Design review of the part built by this model. Coordinates are the model's own, in mm. Give positions to 0.01 mm unless a question says otherwise; leave off trailing zeros. Write each loop counter-clockwise with the first axis right and the second up, starting at its lowest first coordinate (ties: lowest second). Pieces come first, ordered by that corner, then holes.
Autodesk Inventor part; units mm, degrees
ref_plane "YZ Plane" through (0, 0, 0) normal (1, 0, 0) x (0, 1, 0)
ref_plane "XZ Plane" through (0, 0, 0) normal (0, 1, 0) x (-1, 0, 0)
ref_plane "XY Plane" through (0, 0, 0) normal (0, 0, 1) x (1, 0, 0)
sketch "Boceto1" plane through (0, 0, 0) normal (0, 0, 1) x (1, 0, 0)
  line L0 (70, -75) -> (-70, -75)
  line L1 (-70, -75) -> (-70, 75)
  line L2 (-70, 75) -> (70, 75)
  line L3 (70, 75) -> (70, -75)
  line L4 (70, -75) -> (-70, 75) construction
  line L5 (-70, -75) -> (70, 75) construction
  point P0 (0, 0)
  dimension "d0" = 140
  dimension "d1" = 150
extrude "Extrusión1" add sketch "Boceto1" along normal blind 6
sketch "Boceto2" plane through (0, 0, 6) normal (0, 0, 1) x (1, 0, 0)
  line L0 (-70, -75) -> (70, -75)
  line L1 (70, -75) -> (70, 75)
  line L2 (70, 75) -> (-70, 75)
  line L3 (-70, 75) -> (-70, -75)
  line L4 (70, 75) -> (70, 68.9297)
  line L5 (70, 63.9297) -> (70, 57)
  line L6 (70, 53.65) -> (70, 39.3833)
  line L7 (70, 34.3833) -> (70, 20.1167)
  line L8 (70, 16.7667) -> (70, 2.5)
  line L9 (70, -2.5) -> (70, -16.7667)
  line L10 (70, -20.1167) -> (70, -34.3833)
  line L11 (70, 75) -> (70, 68.9297)
  line L12 (61.5, 68.9297) -> (61.5, 63.9297)
  line L13 (70, 63.9297) -> (70, 57)
  line L14 (70, 53.65) -> (70, 39.3833)
  line L15 (70, 34.3833) -> (70, 20.1167)
  line L16 (70, 16.7667) -> (70, 2.5)
  line L17 (61.5, 2.5) -> (61.5, -2.5)
  line L18 (70, -2.5) -> (70, -16.7667)
  line L19 (70, -20.1167) -> (70, -34.3833)
  line L20 (61.5, -34.3833) -> (61.5, -39.3833)
  line L21 (61.5, -63.5) -> (61.5, -68.5)
  line L22 (61.5, 68.9297) -> (55.5, 68.9297)
  line L23 (55.5, 68.9297) -> (55.5, 63.9297)
  line L24 (55.5, 63.9297) -> (61.5, 63.9297)
  line L25 (61.5, 63.9297) -> (61.5, 68.9297)
  line L26 (61.5, 34.3833) -> (55.5, 34.3833)
  line L27 (55.5, 34.3833) -> (55.5, 39.3833)
  line L28 (55.5, 39.3833) -> (61.5, 39.3833)
  line L29 (61.5, 39.3833) -> (61.5, 34.3833)
  line L30 (55.5, 2.5) -> (61.5, 2.5)
  line L31 (61.5, 2.5) -> (61.5, -2.5)
  line L32 (61.5, -2.5) -> (55.5, -2.5)
  line L33 (55.5, -2.5) -> (55.5, 2.5)
  line L34 (55.5, -34.3833) -> (61.5, -34.3833)
  line L35 (61.5, -34.3833) -> (61.5, -39.3833)
  line L36 (61.5, -39.3833) -> (55.5, -39.3833)
  line L37 (55.5, -39.3833) -> (55.5, -34.3833)
  line L38 (55.5, -68.5) -> (61.5, -68.5)
  line L39 (61.5, -68.5) -> (61.5, -63.5)
  line L40 (61.5, -63.5) -> (55.5, -63.5)
  line L41 (55.5, -63.5) -> (55.5, -68.5)
  dimension "d7" = 5
  dimension "d8" = 6
  dimension "d9" = 5
  dimension "d12" = 6
  dimension "d16" = 6
  dimension "d35" = 8.5
  dimension "d36" = 6
  dimension "d37" = 8.5
  dimension "d40" = 8.5
  dimension "d45" = 8.5
  dimension "d46" = 8.5
  dimension "d47" = 6
  dimension "d48" = 5
  dimension "d49" = 5
  dimension "d50" = 5
extrude "Extrusión2" cut sketch "Boceto2" against normal blind 6 contours L12 L24 L23 L22 | L17 L32 L33 L30 | L20 L36 L37 L34 | L21 L38 L41 L40 | L26 L27 L28 L29
mirror "Simetría1" about plane through (0, 0, 0) normal (1, 0, 0) of "Extrusión2"
sketch "Boceto4" plane through (0, 0, 6) normal (0, 0, 1) x (1, 0, 0)
  line L0 (70, 75) -> (70, 68.9297)
  line L1 (70, 68.9297) -> (65, 68.9297)
  line L2 (65, 68.9297) -> (65, 63.9297)
  line L3 (65, 63.9297) -> (70, 63.9297)
  line L4 (70, 63.9297) -> (70, 57)
  line L5 (70, 53.65) -> (70, 39.3833)
  line L6 (70, 39.3833) -> (65, 39.3833)
  line L7 (65, 39.3833) -> (65, 34.3833)
  line L8 (65, 34.3833) -> (70, 34.3833)
  line L9 (70, 34.3833) -> (70, 20.1167)
  line L10 (70, 16.7667) -> (70, 2.5)
  line L11 (70, 2.5) -> (65, 2.5)
  line L12 (65, 2.5) -> (65, -2.5)
  line L13 (65, -2.5) -> (70, -2.5)
  line L14 (70, -2.5) -> (70, -16.7667)
  line L15 (70, -20.1167) -> (70, -34.3833)
  line L16 (70, -34.3833) -> (65, -34.3833)
  line L17 (65, -34.3833) -> (65, -39.3833)
  line L18 (65, -39.3833) -> (70, -39.3833)
  line L19 (70, -39.3833) -> (70, -53.65)
  line L20 (70, -57) -> (70, -63.5)
  line L21 (70, 75) -> (70, 68.9297)
  line L22 (70, 68.9297) -> (65, 68.9297)
  line L23 (65, 68.9297) -> (65, 63.9297)
  line L24 (65, 63.9297) -> (70, 63.9297)
  line L25 (70, 63.9297) -> (70, 57)
  line L26 (70, 57) -> (76.2, 57)
  line L27 (76.2, 57) -> (76.2, 58.3)
  line L28 (76.2, 58.3) -> (79, 58.3)
  line L29 (79, 58.3) -> (79, 57)
  line L30 (79, 57) -> (82, 57)
  line L31 (82, 57) -> (82, 53.65)
  line L32 (82, 53.65) -> (79, 53.65)
  line L33 (79, 53.65) -> (79, 52.35)
  line L34 (79, 52.35) -> (76.2, 52.35)
  line L35 (76.2, 52.35) -> (76.2, 53.65)
  line L36 (76.2, 53.65) -> (70, 53.65)
  line L37 (70, 53.65) -> (70, 39.3833)
  line L38 (70, 39.3833) -> (65, 39.3833)
  line L39 (65, 39.3833) -> (65, 34.3833)
  line L40 (65, 34.3833) -> (70, 34.3833)
  line L41 (70, 34.3833) -> (70, 20.1167)
  line L42 (70, 20.1167) -> (76.2, 20.1167)
  line L43 (76.2, 20.1167) -> (76.2, 21.4167)
  line L44 (76.2, 21.4167) -> (79, 21.4167)
  line L45 (79, 21.4167) -> (79, 20.1167)
  line L46 (79, 20.1167) -> (82, 20.1167)
  line L47 (82, 20.1167) -> (82, 16.7667)
  line L48 (82, 16.7667) -> (79, 16.7667)
  line L49 (79, 16.7667) -> (79, 15.4667)
  line L50 (79, 15.4667) -> (76.2, 15.4667)
  line L51 (76.2, 15.4667) -> (76.2, 16.7667)
  line L52 (76.2, 16.7667) -> (70, 16.7667)
  line L53 (70, 16.7667) -> (70, 2.5)
  line L54 (70, 2.5) -> (65, 2.5)
  line L55 (65, 2.5) -> (65, -2.5)
  line L56 (65, -2.5) -> (70, -2.5)
  line L57 (70, -2.5) -> (70, -16.7667)
  line L58 (70, -16.7667) -> (76.2, -16.7667)
  line L59 (76.2, -16.7667) -> (76.2, -15.4667)
  line L60 (76.2, -15.4667) -> (79, -15.4667)
  line L61 (79, -15.4667) -> (79, -16.7667)
  line L62 (79, -16.7667) -> (82, -16.7667)
  line L63 (82, -16.7667) -> (82, -20.1167)
  line L64 (82, -20.1167) -> (79, -20.1167)
  line L65 (79, -20.1167) -> (79, -21.4167)
  line L66 (79, -21.4167) -> (76.2, -21.4167)
  line L67 (76.2, -21.4167) -> (76.2, -20.1167)
  line L68 (76.2, -20.1167) -> (70, -20.1167)
  line L69 (70, -20.1167) -> (70, -34.3833)
  line L70 (70, -34.3833) -> (65, -34.3833)
  line L71 (65, -34.3833) -> (65, -39.3833)
  line L72 (65, -39.3833) -> (70, -39.3833)
  line L73 (70, -39.3833) -> (70, -53.65)
  line L74 (70, -53.65) -> (76.2, -53.65)
  line L75 (76.2, -53.65) -> (76.2, -52.35)
  line L76 (76.2, -52.35) -> (79, -52.35)
  line L77 (79, -52.35) -> (79, -53.65)
  line L78 (79, -53.65) -> (82, -53.65)
  line L79 (82, -53.65) -> (82, -57)
  line L80 (82, -57) -> (79, -57)
  line L81 (79, -57) -> (79, -58.3)
  line L82 (79, -58.3) -> (76.2, -58.3)
  line L83 (76.2, -58.3) -> (76.2, -57)
  line L84 (76.2, -57) -> (70, -57)
  line L85 (70, -57) -> (70, -63.5)
  line L86 (70, -63.5) -> (65, -63.5)
  line L87 (65, -63.5) -> (65, -68.5)
  line L88 (65, -68.5) -> (70, -68.5)
  line L89 (70, -68.5) -> (70, -75)
  line L90 (70, 75) -> (70, -75)
  line L91 (-61.5, -63.5) -> (-55.5, -63.5)
  line L92 (-55.5, -63.5) -> (-55.5, -68.5)
  line L93 (-55.5, -68.5) -> (-61.5, -68.5)
  line L94 (-61.5, -68.5) -> (-61.5, -63.5)
  line L95 (-61.5, 2.5) -> (-55.5, 2.5)
  line L96 (-55.5, 2.5) -> (-55.5, -2.5)
  line L97 (-55.5, -2.5) -> (-61.5, -2.5)
  line L98 (-61.5, -2.5) -> (-61.5, 2.5)
  line L99 (-61.5, 34.3833) -> (-61.5, 39.3833)
  line L100 (-61.5, 39.3833) -> (-55.5, 39.3833)
  line L101 (-55.5, 39.3833) -> (-55.5, 34.3833)
  line L102 (-55.5, 34.3833) -> (-61.5, 34.3833)
  line L103 (-61.5, -34.3833) -> (-55.5, -34.3833)
  line L104 (-55.5, -34.3833) -> (-55.5, -39.3833)
  line L105 (-55.5, -39.3833) -> (-61.5, -39.3833)
  line L106 (-61.5, -39.3833) -> (-61.5, -34.3833)
  line L107 (-55.5, 68.9297) -> (-55.5, 63.9297)
  line L108 (-55.5, 63.9297) -> (-61.5, 63.9297)
  line L109 (-61.5, 63.9297) -> (-61.5, 68.9297)
  line L110 (-61.5, 68.9297) -> (-55.5, 68.9297)
  line L111 (55.5, -63.5) -> (61.5, -63.5)
  line L112 (61.5, -63.5) -> (61.5, -68.5)
  line L113 (61.5, -68.5) -> (55.5, -68.5)
  line L114 (55.5, -68.5) -> (55.5, -63.5)
  line L115 (55.5, 2.5) -> (61.5, 2.5)
  line L116 (61.5, 2.5) -> (61.5, -2.5)
  line L117 (61.5, -2.5) -> (55.5, -2.5)
  line L118 (55.5, -2.5) -> (55.5, 2.5)
  line L119 (61.5, 39.3833) -> (61.5, 34.3833)
  line L120 (61.5, 34.3833) -> (55.5, 34.3833)
  line L121 (55.5, 34.3833) -> (55.5, 39.3833)
  line L122 (55.5, 39.3833) -> (61.5, 39.3833)
  line L123 (55.5, -34.3833) -> (61.5, -34.3833)
  line L124 (61.5, -34.3833) -> (61.5, -39.3833)
  line L125 (61.5, -39.3833) -> (55.5, -39.3833)
  line L126 (55.5, -39.3833) -> (55.5, -34.3833)
  line L127 (55.5, 63.9297) -> (55.5, 68.9297)
  line L128 (55.5, 68.9297) -> (61.5, 68.9297)
  line L129 (61.5, 68.9297) -> (61.5, 63.9297)
  line L130 (61.5, 63.9297) -> (55.5, 63.9297)
  line L131 (-70, -75) -> (70, -75)
  line L132 (70, -75) -> (70, 75)
  line L133 (70, 75) -> (-70, 75)
  line L134 (-70, 75) -> (-70, -75)
  circle A0 centre (58.5, 55.325) radius 2.5
  circle A1 centre (58.5, 18.4417) radius 2.5
  circle A2 centre (58.5, -17.8117) radius 2.5
  circle A3 centre (58.5, -55.325) radius 2.5
  line L135 (55.5, -63.5) -> (61.5, -63.5)
  point P0 (58.5, -63.5)
  point P1 (58.5, -63.5)
  point P2 (58.5, -63.5)
  point P3 (58.5, 2.5)
  point P4 (58.5, 39.3833)
  dimension "d28" = 5
  dimension "d29" = 5
  dimension "d30" = 5
  dimension "d31" = 5
extrude "Extrusión4" cut sketch "Boceto4" against normal blind 6 contours A0 | A1 | A2 | A3
mirror "Simetría3" about plane through (0, 0, 0) normal (1, 0, 0) of "Extrusión4"
sketch "Boceto5" plane through (0, 0, 6) normal (0, 0, 1) x (1, 0, 0)
  circle A0 centre (-8.2, 15) radius 1.6
  line L0 (70, 75) -> (-70, 75)
  line L1 (-70, 75) -> (-70, -75)
  line L2 (-70, -75) -> (-70, 75)
  circle A1 centre (26.8, -35) radius 3.6
  point P0 (0, 0)
  dimension "d51" = 60
  dimension "d52" = 3.2
  dimension "d53" = 61.8
  dimension "d63" = 7.2
  dimension "d64" = 35
  dimension "d65" = 50
extrude "Extrusión5" cut sketch "Boceto5" against normal blind 6 contours A0
extrude "Extrusión7" cut sketch "Boceto5" against normal blind 6 contours A1
sketch "Boceto6" plane through (0, 0, 6) normal (0, 0, 1) x (1, 0, 0)
  circle A0 centre (26.8, -35) radius 3.6
  line L0 (4.8, -35) -> (48.8, -35)
  circle A1 centre (4.8, -35) radius 1.5
  circle A2 centre (48.8, -35) radius 1.5
  point P0 (0, 0)
  dimension "d68" = 44
  dimension "d69" = 3
  dimension "d70" = 3
extrude "Extrusión8" cut sketch "Boceto6" against normal blind 6 contours A1 | A2
properties part number "Plano 2" material "Vidrio"
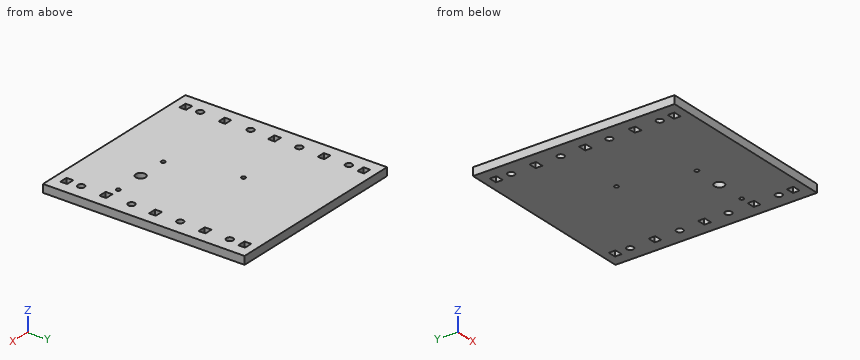
(1) Consider section A-A, the plane y = 66. Give the boundary of the cut face in (x, z), then the cut area to 3 significant figures.
Resolved:
outline: (-70, 0) - (-61.5, 0) - (-61.5, 6) - (-70, 6) - close; (-55.5, 0) - (55.5, 0) - (55.5, 6) - (-55.5, 6) - close; (61.5, 0) - (70, 0) - (70, 6) - (61.5, 6) - close
area: 768 mm2
(2) Clearance check with flat-ended pins moving along their axes: P1, Ø11.5, axis at x = 26.8, y = -35, coming from the -Z side; P2, Ø2.5, axis at x = 4.8, y = -35, coming from the -Z side. State where each tip first meets the part, or that it passes through.
Resolved:
P1: stops at z = 0
P2: passes through
(3) Consider section B-B, the plane x = 58.5. Give the number of separate pieces and of enclosed holes in the cut face, then the cut area to 3 significant figures.
Resolved:
separate pieces: 10
enclosed holes: 0
area: 630 mm2
(4) To check wall thickness, follow L1, parallel to X at y = 36, z = 2.7; L2, parallel to Y at x = -8.2, z = 2; L3, parallel to X at y = -38, z = 3.75. State the ranges of each line that lie inside material, in increasing order.
Resolved:
L1: x = -70 to -61.5, -55.5 to 55.5, 61.5 to 70
L2: y = -75 to 13.4, 16.6 to 75
L3: x = -70 to -61.5, -55.5 to 24.81, 28.79 to 55.5, 61.5 to 70
